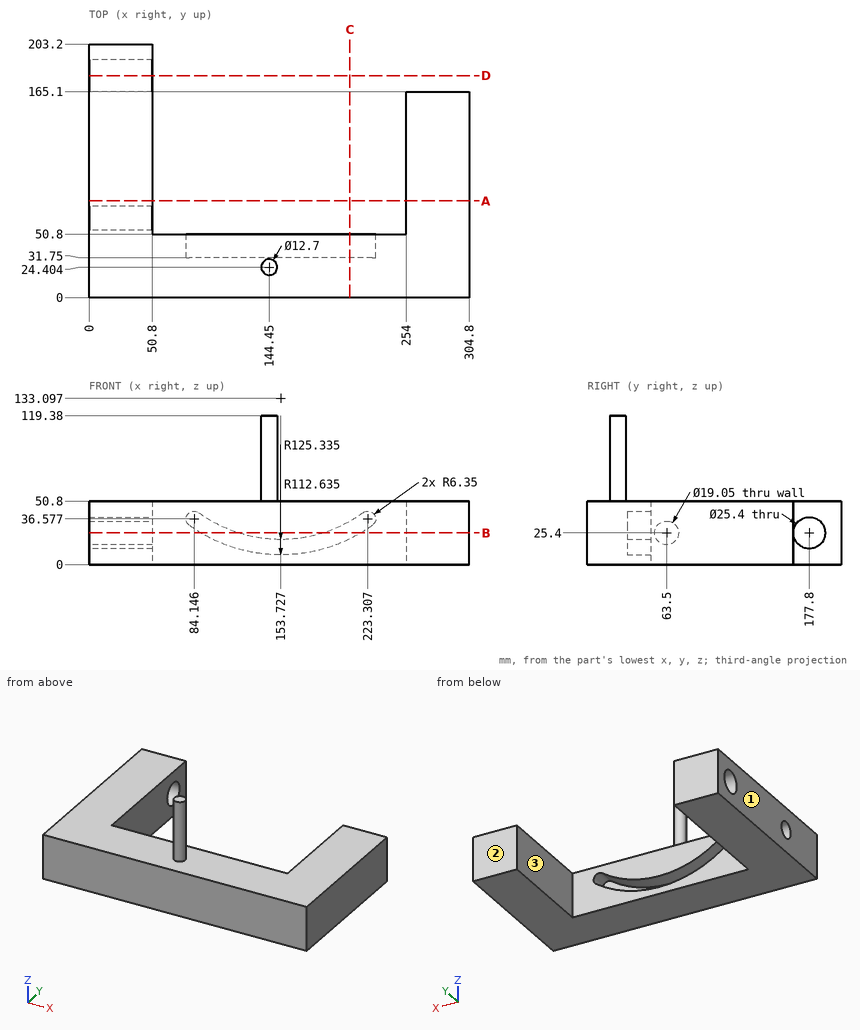
The figure shows three views and two pictorial views of one solid part (mm, origin at its lowest corner). Answer the questions. A direction names the side the tool comes from. Give positions to 0.01 mm unless a question says otherwise; leave off trailing zeros. Write each loop counter-clockwise with the first axis right and the second up, starting at its lowest first coordinate (ties: lowest second). Pieces come first, ordered by that corner, then holes. Notation, with made-up numbers: (4, 3) - (32, 3) arc R29 ccw to (32, 42) - close; hole circle Ø6 at (72, -27.75). An arc over 180 degrees is marked (long way). Use one line per item in the form item = value. Start each with the question number.
1) Find section D-D on y = 177.8. Determine the outline of the cut face in (x, z), plus the area to 3 significant figures.
2) Find section A-A on y = 77.5. Determine the outline of the cut face in (x, z), plus the area to 3 significant figures.
3) A tool of negligible diameter and unlimited length cuts with its end or side. For the marked faces 1, 2 and 3, from which of +Z, -Z, +X, -X, +Y, -Y can it reach the whole face along a straight path? Write none if from no direction.
4) Flat-ended cylindrical pins translate along their axes: pin 1 Ø4 at (x, y) = (263.5, 54.5) entering from +Z; pin 2 Ø8 at (x, z) = (141, 68) entering from -Y; pin 3 Ø15 at (x, z) = (164.5, 25.5) entering from +Y. Find the tip coordinate at first contact, or state that the pin passes through.
5) Consider line 1 along Y through (x, z) = (28.5, 25.4) (1 decimal); line 2 along Z through (x, y) = (17, 177) (1 decimal); line 3 along Y through (x, z) = (46, 18) (1 decimal). Determine where each line is inside the solid, lowest interval first. Write a range as from..to.
6) Find section B-B on z = 25.4. Count the separate pieces of the cut face and the enclosed holes in it, plus the area to 3 significant figures.
7) Find section C-C on x = 209. Determine the outline of the cut face in (y, z).
Geometry results:
q1.outline = (0, 0) - (50.8, 0) - (50.8, 12.7) - (0, 12.7) - close; (0, 38.1) - (50.8, 38.1) - (50.8, 50.8) - (0, 50.8) - close
q1.area = 1,290 mm2
q2.outline = (0, 0) - (50.8, 0) - (50.8, 50.8) - (0, 50.8) - close; (254, 0) - (304.8, 0) - (304.8, 50.8) - (254, 50.8) - close
q2.area = 5,160 mm2
q3.face_1 = +Z, -Z, -X, +Y, -Y
q3.face_2 = +Z, -Z, +X, +Y
q3.face_3 = +Z, -Z, +Y
q4.pin_1 = 50.8
q4.pin_2 = 18.05
q4.pin_3 = 50.8
q5.line_1 = 0..54, 73..165.1, 190.5..203.2
q5.line_2 = 0..12.7, 38.1..50.8
q5.line_3 = 0..57.5, 69.5..167.5, 188.1..203.2
q6.separate_pieces = 3
q6.enclosed_holes = 0
q6.area = 25,600 mm2
q7.outline = (0, 0) - (50.8, 0) - (50.8, 20.61) - (31.75, 20.61) - (31.75, 34.96) - (50.8, 34.96) - (50.8, 50.8) - (0, 50.8) - close
